Work out the finished part from the listing and answer in its coordinate system (mm). A direction names the side the tool comes from. Round coordinates to 2 decimals unless told otherwise and drop trailing zeros. Loops run counter-clockwise (first coordinate to the right, second up) from the corner with the lowest first, then second, coordinate; pieces in that order, holes last. Notation, with made-up numbers: (9.5, -26.5) - (35.5, -26.5) arc R23 cw to (35.5, -8.5) - close; hole circle Ø1 at (-0.75, 41). An arc over 180 degrees is marked (long way). Return JSON: item names as keys, results as strings.
from build123d import *

# Parameters (mm, degrees)
SKETCH_1_W          = 145
SKETCH_1_H          = 145
SKETCH_1_R          = 38.7
SKETCH_1_R_2        = 2
EXTRUDE_1_DEPTH     = 4
SKETCH_2_OUTSIDE_W  = 188.02
SKETCH_2_OUTSIDE_H  = 188.02
SKETCH_2_OUTSIDE_R  = 61
CUT_EXTRUDE_1_DEPTH = 0.1
SKETCH_3_R          = 1.25
EXTRUDE_2_DEPTH     = 4
SKETCH_5_R          = 2
CUT_EXTRUDE_2_DEPTH = 4
SKETCH_7_R          = 47.5
SKETCH_7_W          = 32
SKETCH_7_H          = 7.011387078
SKETCH_7_H_2        = 7
CUT_EXTRUDE_4_DEPTH = 4
SKETCH_8_W          = 15
SKETCH_8_H          = 6
EXTRUDE_3_DEPTH     = 4
FILLET_4_R          = 10
CUT_EXTRUDE_6_DEPTH = 4
EXTRUDE_5_DEPTH     = 4
CUT_EXTRUDE_7_DEPTH = 4
CUT_EXTRUDE_8_DEPTH = 4


with BuildPart() as part:
    # 草图1 → 凸台-拉伸1 (new body)
    with BuildSketch(Plane.XY):
        Rectangle(SKETCH_1_W, SKETCH_1_H)
        Circle(SKETCH_1_R, mode=Mode.SUBTRACT)
        with Locations((16.838071024, 40.65069943)):
            Circle(SKETCH_1_R_2, mode=Mode.SUBTRACT)
        with Locations((40.65069943, 16.838071024)):
            Circle(SKETCH_1_R_2, mode=Mode.SUBTRACT)
        with Locations((40.65069943, -16.838071024)):
            Circle(SKETCH_1_R_2, mode=Mode.SUBTRACT)
        with Locations((16.838071024, -40.65069943)):
            Circle(SKETCH_1_R_2, mode=Mode.SUBTRACT)
        with Locations((-16.838071024, -40.65069943)):
            Circle(SKETCH_1_R_2, mode=Mode.SUBTRACT)
        with Locations((-40.65069943, -16.838071024)):
            Circle(SKETCH_1_R_2, mode=Mode.SUBTRACT)
        with Locations((-40.65069943, 16.838071024)):
            Circle(SKETCH_1_R_2, mode=Mode.SUBTRACT)
        with Locations((-16.838071024, 40.65069943)):
            Circle(SKETCH_1_R_2, mode=Mode.SUBTRACT)
    extrude(amount=EXTRUDE_1_DEPTH)

    # 草图2 outside → 切除-拉伸1 (cut)
    with BuildSketch(Plane.XY.offset(4)):
        Rectangle(SKETCH_2_OUTSIDE_W, SKETCH_2_OUTSIDE_H)
        Circle(SKETCH_2_OUTSIDE_R, mode=Mode.SUBTRACT)
    extrude(amount=-CUT_EXTRUDE_1_DEPTH, mode=Mode.SUBTRACT)

    # 草图3 → 凸台-拉伸2 (add)
    # profile 1 of 2: a face of its own
    with BuildSketch(Plane(origin=(0, 0, 0), x_dir=(-1, 0, 0), z_dir=(0, 0, -1))):
        with BuildLine():
            Line((79.5, -72.5), (97.5, -72.5))
            Line((97.5, -72.5), (97.5, -45.069390943))
            ThreePointArc((97.5, -45.069390943), (83.330748854, -37.488728807), (72.5, -25.617376915))
            Line((72.5, -25.617376915), (72.5, -65.5))
            Line((72.5, -65.5), (79.5, -65.5))
            Line((79.5, -65.5), (79.5, -72.5))
        make_face()
        with Locations((84.154569054, -50)):
            Circle(SKETCH_3_R, mode=Mode.SUBTRACT)
        with Locations((92.154569054, -50)):
            Circle(SKETCH_3_R, mode=Mode.SUBTRACT)
    # profile 2 of 2: a face of its own
    with BuildSketch(Plane(origin=(0, 0, 0), x_dir=(-1, 0, 0), z_dir=(0, 0, -1))):
        with BuildLine():
            ThreePointArc((72.5, 25.617376915), (83.330748854, 37.488728807), (97.5, 45.069390943))
            Line((97.5, 45.069390943), (97.5, 72.5))
            Line((97.5, 72.5), (79.5, 72.5))
            Line((79.5, 72.5), (79.5, 65.5))
            Line((79.5, 65.5), (72.5, 65.5))
            Line((72.5, 65.5), (72.5, 25.617376915))
        make_face()
        with Locations((84.154569054, 50)):
            Circle(SKETCH_3_R, mode=Mode.SUBTRACT)
        with Locations((92.154569054, 50)):
            Circle(SKETCH_3_R, mode=Mode.SUBTRACT)
    extrude(amount=-EXTRUDE_2_DEPTH)

    # 草图5 → 切除-拉伸2 (cut)
    with BuildSketch(Plane(origin=(0, 0, 0), x_dir=(-1, 0, 0), z_dir=(0, 0, -1))):
        with Locations((-67.5, 41.5)):
            Circle(SKETCH_5_R)
        with Locations((-41.5, 67.5)):
            Circle(SKETCH_5_R)
        with Locations((-51.5, 67.5)):
            Circle(SKETCH_5_R)
        with Locations((-51.5, 57.5)):
            Circle(SKETCH_5_R)
        with Locations((-41.5, 57.5)):
            Circle(SKETCH_5_R)
        with Locations((-57.5, 41.5)):
            Circle(SKETCH_5_R)
        with Locations((-57.5, 51.5)):
            Circle(SKETCH_5_R)
        with Locations((-67.5, 51.5)):
            Circle(SKETCH_5_R)
        with Locations(Location((67.5, 51.5, 0), (0, 0, 180))):
            Circle(SKETCH_5_R)
        with Locations(Location((57.5, 51.5, 0), (0, 0, 180))):
            Circle(SKETCH_5_R)
        with Locations(Location((57.5, 41.5, 0), (0, 0, 180))):
            Circle(SKETCH_5_R)
        with Locations(Location((41.5, 57.5, 0), (0, 0, 180))):
            Circle(SKETCH_5_R)
        with Locations(Location((51.5, 57.5, 0), (0, 0, 180))):
            Circle(SKETCH_5_R)
        with Locations(Location((51.5, 67.5, 0), (0, 0, 180))):
            Circle(SKETCH_5_R)
        with Locations(Location((41.5, 67.5, 0), (0, 0, 180))):
            Circle(SKETCH_5_R)
        with Locations(Location((67.5, 41.5, 0), (0, 0, 180))):
            Circle(SKETCH_5_R)
        with Locations((67.5, -41.5)):
            Circle(SKETCH_5_R)
        with Locations((41.5, -67.5)):
            Circle(SKETCH_5_R)
        with Locations((51.5, -67.5)):
            Circle(SKETCH_5_R)
        with Locations((51.5, -57.5)):
            Circle(SKETCH_5_R)
        with Locations((41.5, -57.5)):
            Circle(SKETCH_5_R)
        with Locations((57.5, -41.5)):
            Circle(SKETCH_5_R)
        with Locations((57.5, -51.5)):
            Circle(SKETCH_5_R)
        with Locations((67.5, -51.5)):
            Circle(SKETCH_5_R)
        with Locations(Location((-67.5, -51.5, 0), (0, 0, 180))):
            Circle(SKETCH_5_R)
        with Locations(Location((-57.5, -51.5, 0), (0, 0, 180))):
            Circle(SKETCH_5_R)
        with Locations(Location((-57.5, -41.5, 0), (0, 0, 180))):
            Circle(SKETCH_5_R)
        with Locations(Location((-41.5, -57.5, 0), (0, 0, 180))):
            Circle(SKETCH_5_R)
        with Locations(Location((-51.5, -57.5, 0), (0, 0, 180))):
            Circle(SKETCH_5_R)
        with Locations(Location((-51.5, -67.5, 0), (0, 0, 180))):
            Circle(SKETCH_5_R)
        with Locations(Location((-41.5, -67.5, 0), (0, 0, 180))):
            Circle(SKETCH_5_R)
        with Locations(Location((-67.5, -41.5, 0), (0, 0, 180))):
            Circle(SKETCH_5_R)
    extrude(amount=-CUT_EXTRUDE_2_DEPTH, mode=Mode.SUBTRACT)

    # 草图7 → 切除-拉伸4 (cut)
    with BuildSketch(Plane(origin=(0, 0, 0), x_dir=(-1, 0, 0), z_dir=(0, 0, -1))):
        with Locations((112.5, 0)):
            Circle(SKETCH_7_R)
        with Locations((81.5, 68.994306461)):
            Rectangle(SKETCH_7_W, SKETCH_7_H)
        with Locations((81.5, -69)):
            Rectangle(SKETCH_7_W, SKETCH_7_H_2)
    extrude(amount=-CUT_EXTRUDE_4_DEPTH, mode=Mode.SUBTRACT)

    # 草图8 → 凸台-拉伸3 (add)
    with BuildSketch(Plane(origin=(0, 0, 0), x_dir=(-1, 0, 0), z_dir=(0, 0, -1))):
        with Locations((90, 68.488612922)):
            Rectangle(SKETCH_8_W, SKETCH_8_H)
    extrude_3 = extrude(amount=-EXTRUDE_3_DEPTH)

    # 镜向1: 凸台-拉伸3 across plane
    add(extrude_3.mirror(Plane.ZX))

    # 圆角4
    fillet_4_edges = [part.edges().sort_by_distance(p)[0] for p in [
        (72.5, -72.5, 1.95),
        (72.5, 72.5, 1.95),
    ]]
    fillet(fillet_4_edges, radius=FILLET_4_R)

    # 草图12 → 切除-拉伸6 (cut)
    with BuildSketch(Plane(origin=(0, 0, 0), x_dir=(-1, 0, 0), z_dir=(0, 0, -1))):
        with BuildLine():
            Line((84.154569054, 47.5), (77.154569054, 47.5))
            ThreePointArc((77.154569054, 47.5), (74.654569054, 50), (77.154569054, 52.5))
            Line((77.154569054, 52.5), (84.154569054, 52.5))
            ThreePointArc((84.154569054, 52.5), (86.654569054, 50), (84.154569054, 47.5))
        make_face()
        with BuildLine():
            Line((84.154569054, -52.5), (77.154569054, -52.5))
            ThreePointArc((77.154569054, -52.5), (74.654569054, -50), (77.154569054, -47.5))
            Line((77.154569054, -47.5), (84.154569054, -47.5))
            ThreePointArc((84.154569054, -47.5), (86.654569054, -50), (84.154569054, -52.5))
        make_face()
    extrude(amount=-CUT_EXTRUDE_6_DEPTH, mode=Mode.SUBTRACT)

    # 草图13 → 凸台-拉伸5 (add)
    with BuildSketch(Plane(origin=(0, 0, 0), x_dir=(-1, 0, 0), z_dir=(0, 0, -1))):
        with BuildLine():
            Line((97.5, -71.488612922), (142.5, -71.488612922))
            Line((142.5, -71.488612922), (142.5, -32.5))
            Line((142.5, -32.5), (112.5, -32.5))
            ThreePointArc((112.5, -32.5), (80, 0), (112.5, 32.5))
            Line((112.5, 32.5), (142.5, 32.5))
            Line((142.5, 32.5), (142.5, 71.488612922))
            Line((142.5, 71.488612922), (97.5, 71.488612922))
            Line((97.5, 71.488612922), (97.5, 45.069390943))
            ThreePointArc((97.5, 45.069390943), (65, 0), (97.5, -45.069390943))
            Line((97.5, -45.069390943), (97.5, -71.488612922))
        make_face()
    extrude(amount=-EXTRUDE_5_DEPTH)

    # 草图14 → 切除-拉伸7 (cut)
    with BuildSketch(Plane(origin=(0, 0, 0), x_dir=(-1, 0, 0), z_dir=(0, 0, -1))):
        with BuildLine():
            Line((97.566987559, 52.5), (104.566987559, 52.5))
            ThreePointArc((104.566987559, 52.5), (107.066987559, 50), (104.566987559, 47.5))
            Line((104.566987559, 47.5), (97.566987559, 47.5))
            ThreePointArc((97.566987559, 47.5), (95.066987559, 50), (97.566987559, 52.5))
        make_face()
        with BuildLine():
            Line((122.566987559, 52.5), (129.566987559, 52.5))
            ThreePointArc((129.566987559, 52.5), (132.066987559, 50), (129.566987559, 47.5))
            Line((129.566987559, 47.5), (122.566987559, 47.5))
            ThreePointArc((122.566987559, 47.5), (120.066987559, 50), (122.566987559, 52.5))
        make_face()
        with BuildLine():
            Line((122.566987559, -52.5), (129.566987559, -52.5))
            ThreePointArc((129.566987559, -52.5), (132.066987559, -50), (129.566987559, -47.5))
            Line((129.566987559, -47.5), (122.566987559, -47.5))
            ThreePointArc((122.566987559, -47.5), (120.066987559, -50), (122.566987559, -52.5))
        make_face()
        with BuildLine():
            Line((97.566987559, -52.5), (104.566987559, -52.5))
            ThreePointArc((104.566987559, -52.5), (107.066987559, -50), (104.566987559, -47.5))
            Line((104.566987559, -47.5), (97.566987559, -47.5))
            ThreePointArc((97.566987559, -47.5), (95.066987559, -50), (97.566987559, -52.5))
        make_face()
    extrude(amount=-CUT_EXTRUDE_7_DEPTH, mode=Mode.SUBTRACT)

    # 草图16 → 切除-拉伸8 (cut)
    with BuildSketch(Plane(origin=(0, 0, 0), x_dir=(-1, 0, 0), z_dir=(0, 0, -1))):
        with BuildLine():
            Line((73.566987559, 22.5), (80.566987559, 22.5))
            ThreePointArc((80.566987559, 22.5), (83.066987559, 20), (80.566987559, 17.5))
            Line((80.566987559, 17.5), (73.566987559, 17.5))
            ThreePointArc((73.566987559, 17.5), (71.066987559, 20), (73.566987559, 22.5))
        make_face()
        with BuildLine():
            Line((73.566987559, -22.5), (80.566987559, -22.5))
            ThreePointArc((80.566987559, -22.5), (83.066987559, -20), (80.566987559, -17.5))
            Line((80.566987559, -17.5), (73.566987559, -17.5))
            ThreePointArc((73.566987559, -17.5), (71.066987559, -20), (73.566987559, -22.5))
        make_face()
    extrude(amount=-CUT_EXTRUDE_8_DEPTH, mode=Mode.SUBTRACT)


solid = part.part
1) Flat-ended cylindrical pins translate along their axes: pin 1 (2.5 mm diameter, centred on x = -67.5, y = 51.5, fed in from -Z); pin 2 (4.5 mm diameter, centred on x = -51.5, y = -57.5, fed in from +Z). Find the tip coordinate at first contact, or state that the pin passes through.
Verdict:
{"pin 1": "passes through", "pin 2": "stops at z = 3.9"}
2) Find the intervals of material crossed by L1, parallel to Y at x = 51.5, z = 1.4; L2, parallel to Y at x = -57.5, z = 1.7; L3, parallel to Y at x = -133.5, z = 3.85, in increasing order.
Verdict:
{"L1": "y = -72.5 to -69.5, -65.5 to -59.5, -55.5 to 55.5, 59.5 to 65.5, 69.5 to 72.5", "L2": "y = -72.5 to -53.5, -49.5 to -43.5, -39.5 to 39.5, 43.5 to 49.5, 53.5 to 72.5", "L3": "y = -71.49 to -32.5, 32.5 to 71.49"}
3) Section D-D (z = 1.25) is taken. Count the separate pieces of the cut face and the enclosed holes in it, and give its area (3 significant figures).
Verdict:
{"separate pieces": "1", "enclosed holes": "51", "area": "21,500 mm2"}
4) Section B-B (x = 2) is taken. Give the vertices of the cut face in (y, z).
Verdict:
{"outline": "(-72.5, 0) - (-38.65, 0) - (-38.65, 4) - (-60.97, 4) - (-60.97, 3.9) - (-72.5, 3.9) - close; (38.65, 0) - (72.5, 0) - (72.5, 3.9) - (60.97, 3.9) - (60.97, 4) - (38.65, 4) - close"}
5) A tool of negligible diameter and unlimited length cuts with its end or side. For faces 5 (the flat face through (-65.5, -69, 2)), 6 (the flat face through (-81, -47.5, 2)), from which of +Z, -Z, +X, -X, +Y, -Y can it reach the whole face along a straight path? Write none if from no direction.
Verdict:
{"face 5": "+Z, -Z, -Y", "face 6": "+Z, -Z"}
6) Section C-C (x = 31) is taken. Give the vertices of the cut face in (y, z).
Verdict:
{"outline": "(-72.5, 0) - (-23.17, 0) - (-23.17, 4) - (-52.54, 4) - (-52.54, 3.9) - (-72.5, 3.9) - close; (23.17, 0) - (72.5, 0) - (72.5, 3.9) - (52.54, 3.9) - (52.54, 4) - (23.17, 4) - close"}
7) Section A-A (y = 0) is taken. Give the vertices of the cut face in (x, z).
Verdict:
{"outline": "(-80, 0) - (-38.7, 0) - (-38.7, 4) - (-61, 4) - (-61, 3.9) - (-65, 3.9) - (-65, 4) - (-80, 4) - close; (38.7, 0) - (72.5, 0) - (72.5, 3.9) - (61, 3.9) - (61, 4) - (38.7, 4) - close"}
8) Determine the mould class of faces 1 (the cylindrical face through (69.49, -69.65, 1.98)), 2 (the cylindrical face through (-71.068, 19.945, 1.972)), 3 (the cylindrical face through (-80.008, -0.715, 1.972)), 4 (the cylindrical face through (-41.24, -55.517, 1.923)) for opening direction X: pulls with the +X half, pulls with the -X half, needs draft (parallel to the pull), parting line crosses it, or undercut.
Verdict:
{"face 1": "pulls with the +X half", "face 2": "undercut", "face 3": "pulls with the -X half", "face 4": "undercut"}
